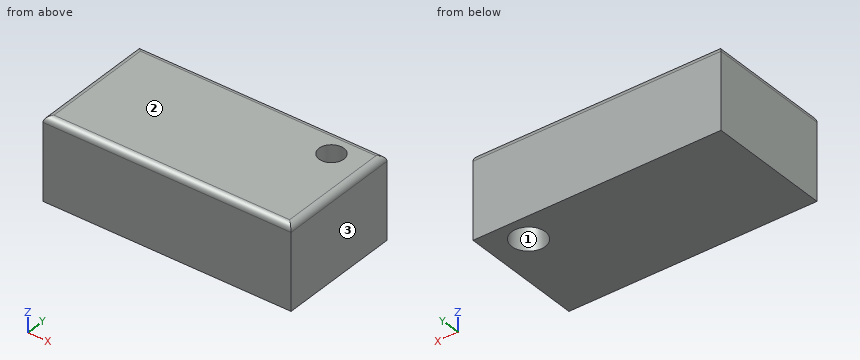
```python
from build123d import *

# Parameters (mm, degrees)
F0_W     = 200
F0_H     = 100
F1_DEPTH = 66.47978
F2_R     = 10
F3_DEPTH = 66.48078
F3_TAPER = -3
F4_R     = 5


with BuildPart() as f1:
    # F0 (on Top) → F1 (new body)
    with BuildSketch(Plane.XY):
        with Locations((100, 50)):
            Rectangle(F0_W, F0_H)
    extrude(amount=F1_DEPTH)

    # F2 (on face) → F3 (cut, through all)
    with BuildSketch(Plane.XY.offset(66.47978)):
        with Locations((171.1803972721, 79.3884024024)):
            Circle(F2_R)
    extrude(amount=-F3_DEPTH, taper=F3_TAPER, mode=Mode.SUBTRACT)

    # F4
    f4_edges = [f1.edges().sort_by_distance(p)[0] for p in [
        (100, 100, 66.47978),
        (100, 0, 66.47978),
        (200, 50, 66.47978),
        (0, 50, 66.47978),
    ]]
    fillet(f4_edges, radius=F4_R)


solid = f1.part
```
For this review, take the finished solid that the model builds, in its own axes (mm). Face numbers are marked on the shaded views. Round coordinates to 2 decimals unless told otherwise and drop trailing zeros. Write each loop counter-clockwise with the first axis right and the second up, starting at its lowest first coordinate (ties: lowest second). Pieces come first, ordered by that corner, then holes.
1) Insertion check: pin 1 Ø6 at (x, y) = (171.5, 44.5) entering from -Z. The pin has a flat end and moves straight along its axis. Give the tip position at first contact, or say it passes through.
Answer below:
pin 1: stops at z = 0
2) Take a section at A-A on z = 40. Give the boundary of the cut face in (x, y).
Answer below:
outline: (0, 0) - (200, 0) - (200, 100) - (0, 100) - close; hole circle Ø22.78 at (171.18, 79.39)
3) For line 1 along X through (y, z) = (75.5, 48); line 2 along Y through (x, z) = (169, 30); line 3 along X through (y, z) = (51.5, 63.5), list the stretches that pass through material, from the lowest coordinate up.
Answer below:
line 1: x = 0 to 160.92, 181.44 to 200
line 2: y = 0 to 67.68, 91.1 to 100
line 3: x = 0.43 to 199.57
4) Take a section at B-B on z = 55. Give the boundary of the cut face in (x, y).
Answer below:
outline: (0, 0) - (200, 0) - (200, 100) - (0, 100) - close; hole circle Ø21.2 at (171.18, 79.39)
5) Mouldability with a two-part tool opening along X and no side actions: class the marked faces 1, 2 and 3 as +X half, -X half, draft (parallel to the pull), parting line (faces both ways), or undercut.
Answer below:
face 1: undercut
face 2: draft
face 3: +X half
